Verification items for this drawing (mm, ordinates from the low corner). Round coordinates to 2 decimals unless told otherwise and drop trailing zeros. Order: outer loops, then holes, each group sorted by start corner. A loop starts at its lowest first (then second) coordinate and runs counter-clockwise, first axis right, second up. Notation, with made-up numbers: M -38,73 L -3,73 A24 ccw -3,110 Z; hole C -14,20.25 d3. An arc over 180 degrees is marked long. One line per item, written item: value. Start each with the question number.
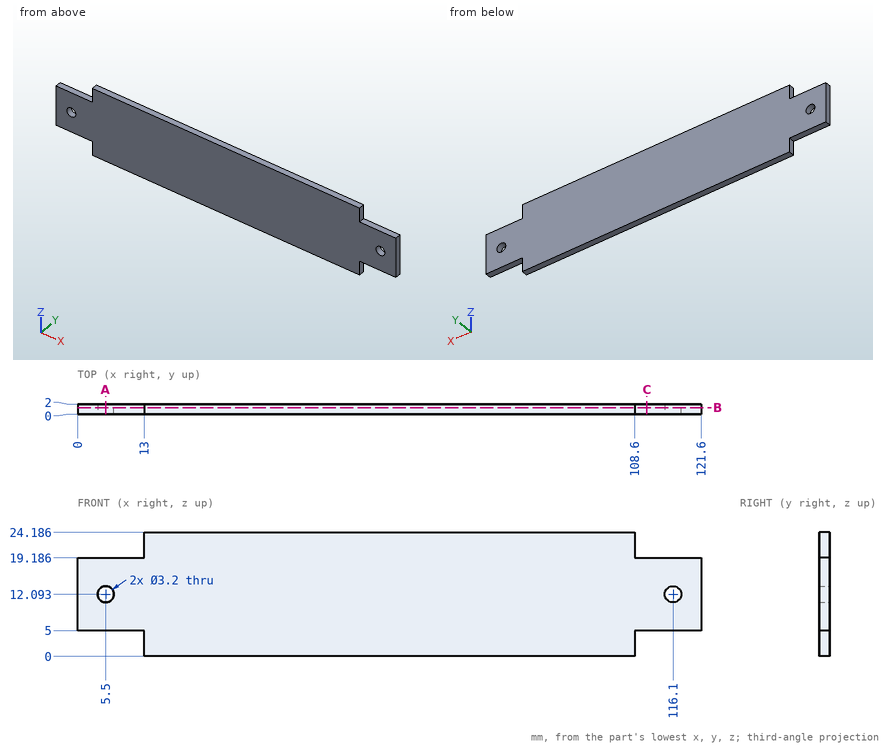
1. Section check B-B (y = 1.3). Record the cut outline in (x, z), and give its area (3 significant figures).
2. Section check C-C (x = 111). Record the cut outline in (y, z).
3. Scan lines: line 1 along X through (y, z) = (0.35, 12.25); line 2 along Z through (x, y) = (5.5, 0.55); line 3 along X through (y, z) = (0.85, 12.75). Record each from-to range of solid material in increasing order.
4. Section check A-A (x = 5.5). Record the cut outline in (y, z), and give its area (3 significant figures).
5. Depth check by flat-ended pin: pin 1 (3 mm diameter, centred on x = 116.1, z = 12.093, fed in from +Y); pin 2 (0.6 mm diameter, centred on y = 1, z = 1.5, fed in from -X); pin 3 (1 mm diameter, centred on y = 1, z = 20.5, fed in from +X). Enter the tip coordinate at first touch or a pass-through.
Geometry check:
1. outline: M 0,5 L 13,5 L 13,0 L 108.6,0 L 108.6,5 L 121.6,5 L 121.6,19.19 L 108.6,19.19 L 108.6,24.19 L 13,24.19 L 13,19.19 L 0,19.19 Z; hole C 5.5,12.09 d3.2; hole C 116.1,12.09 d3.2
1. area: 2,660 mm²
2. outline: M 0,5 L 2,5 L 2,19.19 L 0,19.19 Z
3. line 1: x = 0 to 3.91, 7.09 to 114.51, 117.69 to 121.6
3. line 2: z = 5 to 10.49, 13.69 to 19.19
3. line 3: x = 0 to 4.04, 6.96 to 114.64, 117.56 to 121.6
4. outline: M 0,5 L 2,5 L 2,10.49 L 0,10.49 Z; M 0,13.69 L 2,13.69 L 2,19.19 L 0,19.19 Z
4. area: 22.0 mm²
5. pin 1: passes through
5. pin 2: stops at x = 13
5. pin 3: stops at x = 108.6
